Source: three-view drawing plus pictorial views. Frame: mm from the lowest corner of the part. A direction names the side the tool comes from. Give positions to 0.01 mm unless a question says otherwise; leave off trailing zeros. Write each loop counter-clockwise with the first axis right and the second up, starting at its lowest first coordinate (ties: lowest second). Pieces come first, ordered by that corner, then holes.
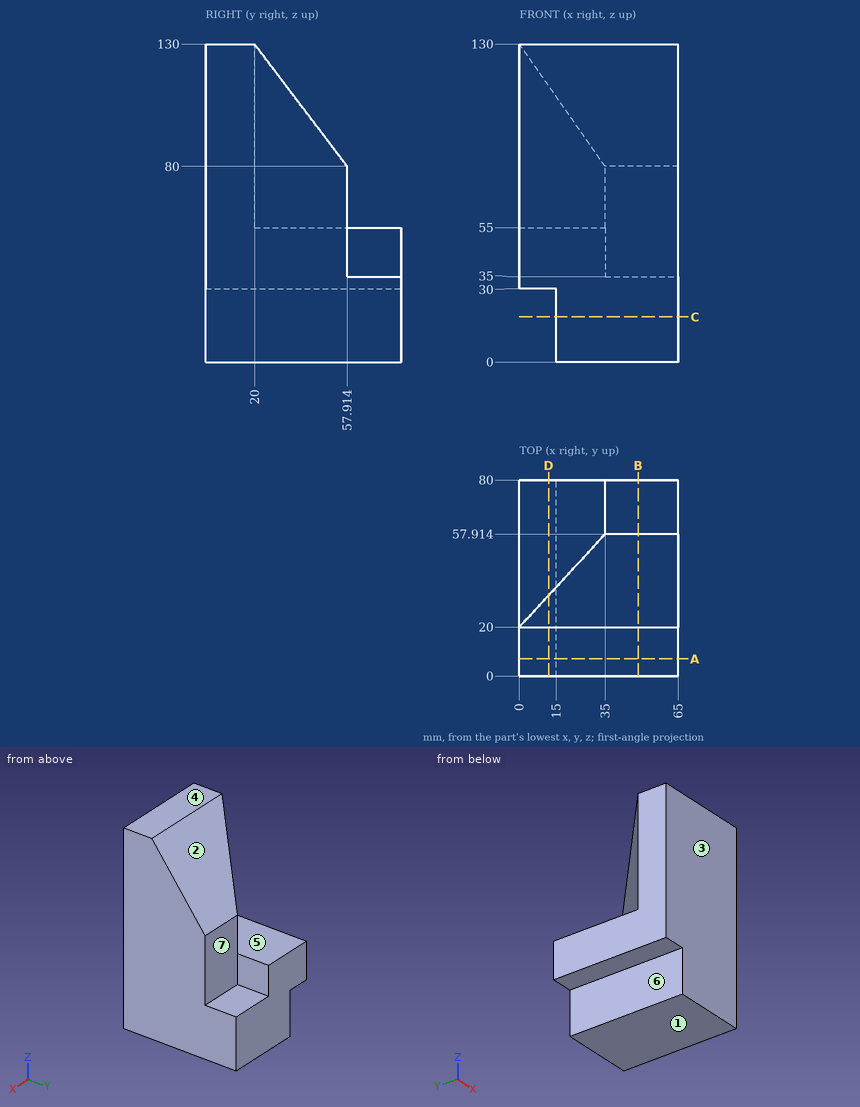
Q1. Section A-A on y = 7. Output: boundary loops of the cut face in (x, z).
Filled sheet:
outline: (0, 30) - (15, 30) - (15, 0) - (65, 0) - (65, 130) - (0, 130) - close
Q2. Section B-B on x = 48.5. Output: boundary loops of the cut face in (y, z), plus the area to 3 significant figures.
Filled sheet:
outline: (0, 0) - (80, 0) - (80, 35) - (57.91, 35) - (57.91, 80) - (20, 130) - (0, 130) - close
area: 7,350 mm2
Q3. Section C-C on z = 18.5. Output: boundary loops of the cut face in (x, y).
Filled sheet:
outline: (15, 0) - (65, 0) - (65, 80) - (15, 80) - close
Q4. Ray query, line 1 along Z through (x, y) = (6, 16); line 2 along Z through (x, y) = (62.5, 70); line 3 along X through (y, z) = (57.5, 27). Return the intervals inside material, ascending.
Filled sheet:
line 1: z = 30 to 130
line 2: z = 0 to 35
line 3: x = 15 to 65
Q5. Access query for the marked faces 4, 5, 6 and 7. Directions: +Z, -Z, +X, -X, +Y, -Y. A direction counts if a zero-diameter tool reaches every point of the face in a straight line with its end or side. Return the directions, or none.
Filled sheet:
face 4: +Z, +X, -X, +Y, -Y
face 5: +Z, -X, +Y
face 6: -Z, -X, +Y, -Y
face 7: +Z, +X, +Y
Q6. Pin query (flat end, axial travel): P1, Ø9, axis at y = 22.5, z = 20, coming from the -X side; P2, Ø9, axis at x = 45.5, z = 55.5, coming from the +Y side; P3, Ø1.5, axis at x = 43, z = 92.5, coming from the +Y side (1 decimal). Return the tip coordinate at first contact, or that it passes through.
Filled sheet:
P1: stops at x = 15
P2: stops at y = 57.91
P3: stops at y = 49
Q7. Pull-direction query (Z, two-part tool) for the marked faces 1, 2 and 3; classes: released by +Z, released by -Z, zero draft, split by the parting line, or undercut.
Filled sheet:
face 1: released by -Z
face 2: released by +Z
face 3: zero draft
Q8. Section D-D on x = 12. Output: boundary loops of the cut face in (y, z), plus the area to 3 significant figures.
Filled sheet:
outline: (0, 30) - (80, 30) - (80, 55) - (33, 55) - (33, 112.86) - (20, 130) - (0, 130) - close
area: 4,360 mm2
